from build123d import *

# Parameters (mm, degrees)
EXTRUDE_1_DEPTH          = 10
SKETCH_2_R               = 30
CUT_EXTRUDE_1_DEPTH      = 15
SKETCH_4_W               = 28
SKETCH_4_H               = 100
EXTRUDE_2_DEPTH          = 20
SKETCH_5_R               = 5
CUT_EXTRUDE_2_DEPTH      = 30
SKETCH_6_R               = 2
CUT_EXTRUDE_4_DEPTH      = 10
PATTERN_CIRCULAR_1_COUNT = 4


with BuildPart() as part:
    # 草图1 → 凸台-拉伸1 (new body)
    with BuildSketch(Plane(origin=(0, 0, 0), x_dir=(1, 0, 0), z_dir=(0, 1, 0))):
        Polygon((0, -50), (125, -50), (125, 50), (-125, 50), (-125, -50), align=None)
    extrude(amount=EXTRUDE_1_DEPTH)

    # 草图2 → 切除-拉伸1 (cut)
    with BuildSketch(Plane(origin=(0, 10, 0), x_dir=(1, 0, 0), z_dir=(0, 1, 0))):
        with Locations(Location((0, 0, 0), (0, 0, 270))):
            Circle(SKETCH_2_R)
    extrude(amount=-CUT_EXTRUDE_1_DEPTH, mode=Mode.SUBTRACT)

    # 草图4 → 凸台-拉伸2 (add)
    with BuildSketch(Plane.XZ):
        with Locations((-111, 0)):
            Rectangle(SKETCH_4_W, SKETCH_4_H)
    extrude_2 = extrude(amount=EXTRUDE_2_DEPTH)

    # 镜向1: 凸台-拉伸2 across plane
    add(extrude_2.mirror(Plane(origin=(0, 0, 0), x_dir=(0, 0, 1), z_dir=(1, 0, 0))))

    # 草图5 → 切除-拉伸2 (cut)
    with BuildSketch(Plane(origin=(125, 0, 0), x_dir=(0, 0, -1), z_dir=(1, 0, 0))):
        with Locations((0, -10)):
            Circle(SKETCH_5_R)
        with Locations((35, -10)):
            Circle(SKETCH_5_R)
        with Locations((-35, -10)):
            Circle(SKETCH_5_R)
    cut_extrude_2 = extrude(amount=-CUT_EXTRUDE_2_DEPTH, mode=Mode.SUBTRACT)

    # 镜向2: 切除-拉伸2 across plane
    add(cut_extrude_2.mirror(Plane(origin=(0, 0, 0), x_dir=(0, 0, 1), z_dir=(1, 0, 0))), mode=Mode.SUBTRACT)

    # 草图6 → 切除-拉伸4 (cut)
    with BuildSketch(Plane(origin=(0, 10, 0), x_dir=(1, 0, 0), z_dir=(0, 1, 0))):
        with Locations(Location((0, 38, 0), (0, 0, 270))):
            Circle(SKETCH_6_R)
    cut_extrude_4 = extrude(amount=-CUT_EXTRUDE_4_DEPTH, mode=Mode.SUBTRACT)

    # 阵列(圆周)1: 切除-拉伸4 ×4 about axis
    pattern_circular_1_axis = Axis((0, 0, 0), (0, 1, 0))
    for i in range(1, PATTERN_CIRCULAR_1_COUNT):
        add(cut_extrude_4.rotate(pattern_circular_1_axis, i * 360 / PATTERN_CIRCULAR_1_COUNT), mode=Mode.SUBTRACT)


solid = part.part
For this review, take the finished solid that the model builds, in its own axes (mm). A direction names the side the tool comes from. Coordinates: 2 decimals unless noted, no trailing zeros. Order: outer loops, then holes, each group sorted by start corner. A loop starts at its lowest first (then second) coordinate and runs counter-clockwise, first axis right, second up. Notation, with made-up numbers: (-4.75, 50) -> (38.25, 50) arc R31 ccw to (38.25, 78) -> close; hole circle Ø3 at (-35.75, 0). An arc over 180 degrees is marked (long way). Return JSON: item names as keys, results as strings.
1. Machinability: for faces 1 (the flat face through (2, 2, -50)), 2 (the flat face through (97, -3, -1)), which of the approach directions +Z, -Z, +X, -X, +Y, -Y give a long, thin tool a straight path to every point of the face, cutting with its end or side? Answer none if there is none.
Answer block:
{"face 1": "-Z, +X, -X, +Y, -Y", "face 2": "+Z, -Z, -Y"}
2. We need section A-A on y = 2.5. Write out the cut boundary in (x, z).
Answer block:
{"outline": "(-125, -50) -> (125, -50) -> (125, 50) -> (-125, 50) -> close; hole circle Ø4 at (-38, 0); hole circle Ø60 at (0, 0); hole circle Ø4 at (0, -38); hole circle Ø4 at (0, 38); hole circle Ø4 at (38, 0)"}
3. For line 1 (Z direction, x = -107.25, y = -10); line 2 (X direction, y = -9.5, z = -18); line 3 (Y direction, x = 113.25, z = 0), list the stretches that pass through material, from the lowest coordinate up. Write a range as from..to.
Answer block:
{"line 1": "-50..-40, -30..-5, 5..30, 40..50", "line 2": "-125..-97, 97..125", "line 3": "-20..-15, -5..10"}
4. For pin 1 Ø6 at (x, z) = (53, -1) entering from -Y; pin 2 Ø3.5 at (x, z) = (0, -38) entering from +Y, all flat-tipped, find the tip position at first contact; note any pin that passes through.
Answer block:
{"pin 1": "y = 0", "pin 2": "through"}
5. We need section D-D on z = 18.5. Write out the cut boundary in (x, y), and give its area (3 significant figures).
Answer block:
{"outline": "(-125, -20) -> (-97, -20) -> (-97, 0) -> (-23.62, 0) -> (-23.62, 10) -> (-125, 10) -> close; (23.62, 0) -> (97, 0) -> (97, -20) -> (125, -20) -> (125, 10) -> (23.62, 10) -> close", "area": "3,150 mm²"}
6. We need section B-B on x = 9.5. Write out the cut boundary in (y, z), and give its area (3 significant figures).
Answer block:
{"outline": "(0, -50) -> (10, -50) -> (10, -28.46) -> (0, -28.46) -> close; (0, 28.46) -> (10, 28.46) -> (10, 50) -> (0, 50) -> close", "area": "431 mm²"}
7. The part is to be moulded in two halves that separate along X. For faces 3 (the flat face through (-23, 0, -23)), 4 (the flat face through (-125, -4.8, -0.7)), 5 (the cylindrical face through (-111.196, -5.043, 0.651)), 6 (the flat face through (125, -4.8, -0.7)), say which applies: +X half, -X half, draft (parallel to the pull), parting line (faces both ways), or undercut.
Answer block:
{"face 3": "undercut", "face 4": "-X half", "face 5": "draft", "face 6": "+X half"}
8. We need section C-C on y = -10. State how many separate pieces and enclosed holes the cut face has, and give its area (3 significant figures).
Answer block:
{"separate pieces": "8", "enclosed holes": "0", "area": "3,920 mm²"}
